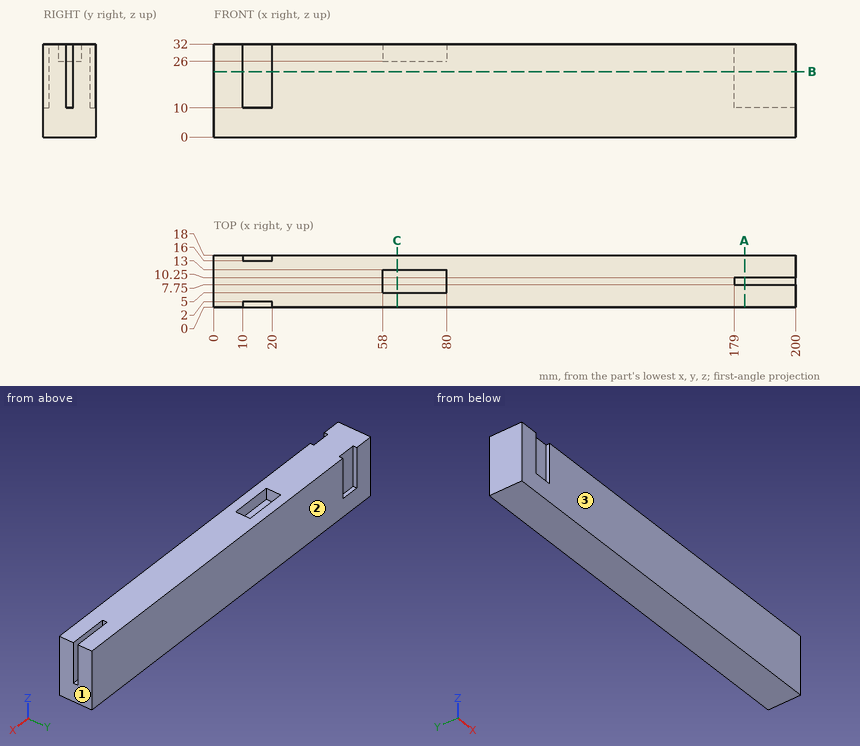
Study the drawing (mm; zero at the part's minimum x, y, z) and answer. Give positions to 0.01 mm unless a question says otherwise; leave off trailing zeros. Loops run counter-clockwise (first coordinate to the right, second up) from the corner with the lowest first, then second, coordinate; pieces in that order, holes last. Notation, with made-up numbers: M 77.25,88.5 L 95.25,88.5 A11 cw 95.25,94.5 Z; hole C 8,87.5 d6. An arc over 180 degrees is marked long. Answer as CSV lines item,"result".
Item 1: The part is cut by section A-A (x = 182.5). Give the vertices of the cut face in (y, z).
Values follow:
outline,"M 0,0 L 18,0 L 18,32 L 10.25,32 L 10.25,10 L 7.75,10 L 7.75,32 L 0,32 Z"
Item 2: The mould has two halves that part along Y. Classify the marked faces 1, 2 and 3: released by +Y, released by -Y, zero draft, split by the parting line, or undercut.
Values follow:
face 1,"zero draft"
face 2,"released by +Y"
face 3,"released by -Y"
Item 3: Given pin 1 Ø1.6 at (x, y) = (13.5, 17.5) entering from +Z; pin 2 Ø1.2 at (y, z) = (9, 25.5) entering from +X; pin 3 Ø3 at (x, z) = (12.5, 16.5) entering from -Y, each flat-ended and moving along its own axis, determine where each tip first touches the part or whether it passes through.
Values follow:
pin 1,"stops at z = 10"
pin 2,"stops at x = 179"
pin 3,"stops at y = 2"
Item 4: Straight lines are drawn through the part: line 1 along X through (y, z) = (9, 30.5); line 2 along X through (y, z) = (16.75, 18.5); line 3 along Y through (x, z) = (187, 10.5). For each, find the intervals that lie inside material, in ascending order. Write a range as [from, to].
Values follow:
line 1,"x = [0, 58], [80, 179]"
line 2,"x = [0, 10], [20, 200]"
line 3,"y = [0, 7.75], [10.25, 18]"
Item 5: The part is cut by section C-C (x = 63). Give the vertices of the cut face in (y, z).
Values follow:
outline,"M 0,0 L 18,0 L 18,32 L 13,32 L 13,26 L 5,26 L 5,32 L 0,32 Z"
Item 6: The part is cut by section B-B (z = 22.5). Give the vertices of the cut face in (x, y).
Values follow:
outline,"M 0,0 L 10,0 L 10,2 L 20,2 L 20,0 L 200,0 L 200,7.75 L 179,7.75 L 179,10.25 L 200,10.25 L 200,18 L 20,18 L 20,16 L 10,16 L 10,18 L 0,18 Z"
